Input: part model. Units: mm. Frame: model coordinates. A direction names the side the tool comes from. Coordinates: 2 decimals unless noted, no trailing zeros. Loops run counter-clockwise (first coordinate to the right, second up) from the corner with the lowest first, then second, coordinate; pieces in that order, holes last. Notation, with made-up numbers: (73.5, 51.25) -> (132.5, 51.25) arc R34 ccw to (132.5, 89.25) -> close; hole circle Ø3 at (0, 34.5). An arc over 180 degrees is marked (long way). Put each result on its own line as item: value. Start each with the question number.
1) Set-up query: faces 1 (the cylindrical face through (-2.58, 4.05, 2.07)), 2 (the cylindrical face through (-7.493, 0.33, 29.732)), 3 (the cylindrical face through (-1.08, -4.88, 15.39)). Return all of +Z, -Z, +X, -X, +Y, -Y with unobstructed straight access to the full face (end or side cutting, diameter ignored); none if empty.
2) Cut plane D-D (x = -4.25). Return the cut outline in (y, z), plus the area to 3 significant figures.
3) Material intervals for L1, parallel to Z at x = -1, y = 4.75; L2, parallel to X at y = 0, z = 5.25, sorted ascending.
4) Contact query for flat-ended pins moving along their axis: P1, Ø5, axis at y = 1.5, z = 14, coming from the +X side; P2, Ø2, axis at x = -3.5, y = 5.5, coming from the -Z side; P3, Ø1, axis at y = 1, z = 4.5, coming from the -X side. Output: stop coordinate, or through.
5) Cut plane A-A (x = 0). Return the cut outline in (y, z).
6) Pull-direction query (X, two-part tool) for faces 4 (the cylindrical face through (0.54, -2.44, 23.4)), 5 (the cylindrical face through (-1.08, -4.88, 0.74)), 6 (the flat face through (2, -2, 0)); classes: pulls with the +X half, pulls with the -X half, needs draft (parallel to the pull), parting line crosses it, or undercut.
7) Cut plane C-C (z = 4). Return the cut outline in (x, y), plus the area to 3 significant figures.
from build123d import *

# Parameters (mm, degrees)
SKIZZE1_R                       = 5
AUFSATZ_LINEAR_AUSTRAGEN1_DEPTH = 31
M6_GEWINDEBOHRUNG1_D            = 5
M6_GEWINDEBOHRUNG1_DEPTH        = 15
M6_GEWINDEBOHRUNG1_TIP          = 1.502151548
M6_GEWINDEBOHRUNG2_D            = 5
M6_GEWINDEBOHRUNG2_DEPTH        = 15
M6_GEWINDEBOHRUNG2_TIP          = 1.502151548
AUFSATZ_LINEAR_START            = -2.5
SKIZZE8_R                       = 7.5
SKIZZE8_R_2                     = 5
AUFSATZ_LINEAR_AUSTRAGEN3_DEPTH = 2.5
SKIZZE9_R                       = 5.404643903
SKIZZE9_R_2                     = 4.8
SCHNITT_LINEAR_AUSTRAGEN1_DEPTH = 1.15


with BuildPart() as part:
    # Skizze1 → Aufsatz-Linear austragen1 (new body)
    with BuildSketch(Plane.XY):
        Circle(SKIZZE1_R)
    extrude(amount=AUFSATZ_LINEAR_AUSTRAGEN1_DEPTH)

    # M6 Gewindebohrung1
    with Locations(Plane(origin=(0, 0, 0), x_dir=(-1, 0, 0), z_dir=(0, 0, -1))):
        with Locations((0, 0)):
            Hole(M6_GEWINDEBOHRUNG1_D / 2, depth=M6_GEWINDEBOHRUNG1_DEPTH)
            with Locations((0, 0, -(M6_GEWINDEBOHRUNG1_DEPTH + M6_GEWINDEBOHRUNG1_TIP / 2))):  # 118° drill point
                Cone(0, M6_GEWINDEBOHRUNG1_D / 2, M6_GEWINDEBOHRUNG1_TIP, mode=Mode.SUBTRACT)

    # M6 Gewindebohrung2
    with Locations(Plane.XY.offset(31)):
        with Locations((0, 0)):
            Hole(M6_GEWINDEBOHRUNG2_D / 2, depth=M6_GEWINDEBOHRUNG2_DEPTH)
            with Locations((0, 0, -(M6_GEWINDEBOHRUNG2_DEPTH + M6_GEWINDEBOHRUNG2_TIP / 2))):  # 118° drill point
                Cone(0, M6_GEWINDEBOHRUNG2_D / 2, M6_GEWINDEBOHRUNG2_TIP, mode=Mode.SUBTRACT)

    # Skizze8 → Aufsatz-Linear austragen3 (add)
    with BuildSketch(Plane.XY.offset(31).offset(AUFSATZ_LINEAR_START)):
        Circle(SKIZZE8_R)
        Circle(SKIZZE8_R_2, mode=Mode.SUBTRACT)
    extrude(amount=AUFSATZ_LINEAR_AUSTRAGEN3_DEPTH)

    # Skizze9 → Schnitt-Linear austragen1 (cut)
    with BuildSketch(Plane(origin=(0, 0, 1.5), x_dir=(-1, 0, 0), z_dir=(0, 0, -1))):
        Circle(SKIZZE9_R)
        Circle(SKIZZE9_R_2, mode=Mode.SUBTRACT)
    extrude(amount=-SCHNITT_LINEAR_AUSTRAGEN1_DEPTH, mode=Mode.SUBTRACT)


solid = part.part
Results found:
1. face 1: none
1. face 2: +Z, -Z
1. face 3: -Z
2. outline: (-6.18, 28.5) -> (-2.63, 28.5) -> (-2.63, 2.65) -> (-2.23, 2.65) -> (-2.23, 1.5) -> (-2.63, 1.5) -> (-2.63, 0) -> (2.63, 0) -> (2.63, 1.5) -> (2.23, 1.5) -> (2.23, 2.65) -> (2.63, 2.65) -> (2.63, 28.5) -> (6.18, 28.5) -> (6.18, 31) -> (-6.18, 31) -> close
2. area: 180 mm2
3. L1: z = 0 to 1.5, 2.65 to 31
3. L2: x = -5 to -2.5, 2.5 to 5
4. P1: stops at x = 5
4. P2: stops at z = 28.5
4. P3: stops at x = -4.97
5. outline: (-7.5, 28.5) -> (-5, 28.5) -> (-5, 2.65) -> (-4.8, 2.65) -> (-4.8, 1.5) -> (-5, 1.5) -> (-5, 0) -> (-2.5, 0) -> (-2.5, 15) -> (-1.67, 15.5) -> (-2.5, 16) -> (-2.5, 31) -> (-7.5, 31) -> close; (1.67, 15.5) -> (2.5, 15) -> (2.5, 0) -> (5, 0) -> (5, 1.5) -> (4.8, 1.5) -> (4.8, 2.65) -> (5, 2.65) -> (5, 28.5) -> (7.5, 28.5) -> (7.5, 31) -> (2.5, 31) -> (2.5, 16) -> close
6. face 4: undercut
6. face 5: parting line crosses it
6. face 6: needs draft
7. outline: circle Ø10 at (0, 0); hole circle Ø5 at (0, 0)
7. area: 58.9 mm2
